from build123d import *

# Parameters (mm, degrees)
BOSS_EXTRU_1_DEPTH      = 5
ESQUISSE12_R            = 3.5
BOSS_EXTRU_2_DEPTH      = 1
ESQUISSE10_RX           = 3.412746185
ESQUISSE10_RY           = 1.923364
ENL_V_MAT_EXTRU_5_DEPTH = 4
ESQUISSE13_R            = 2
ENL_V_MAT_EXTRU_7_DEPTH = 21.846162874
ESQUISSE11_R            = 9.4
ENL_V_MAT_EXTRU_6_DEPTH = 22.060923692


with BuildPart() as part:
    # Esquisse1 → Boss.-Extru.1 (new body)
    with BuildSketch(Plane(origin=(0, 0, 0), x_dir=(1, 0, 0), z_dir=(0, 1, 0))):
        with BuildLine():
            ThreePointArc((-4.625, -8.010734985), (0, -9.25), (4.625, -8.010734985))
            ThreePointArc((4.625, -8.010734985), (9.25, 0), (4.625, 8.010734985))
            ThreePointArc((4.625, 8.010734985), (0, 9.25), (-4.625, 8.010734985))
            ThreePointArc((-4.625, 8.010734985), (-9.25, 0), (-4.625, -8.010734985))
        make_face()
    extrude(amount=BOSS_EXTRU_1_DEPTH)

    # Esquisse8 → Révolution1 (revolve)
    with BuildSketch(Plane.XY, mode=Mode.PRIVATE) as r_volution1_sk:
        Polygon((12.75, 0), (9.25, 0), (9.25, 5), (10.05, 5), align=None)
    revolve(r_volution1_sk.sketch.rotate(Axis((0, 6.978175321, 0), (0, -1, 0)), 90), axis=Axis((0, 6.978175321, 0), (0, -1, 0)))

    # Esquisse12 → Boss.-Extru.2 (add)
    with BuildSketch(Plane.XZ):
        with Locations((0, 12.5)):
            Circle(ESQUISSE12_R)
        with Locations((0, -12.5)):
            Circle(ESQUISSE12_R)
    extrude(amount=-BOSS_EXTRU_2_DEPTH)

    # Esquisse10 → Enlèv. mat.-Extru.5 (cut)
    with BuildSketch(Plane(origin=(0, 5, 0), x_dir=(1, 0, 0), z_dir=(0, 1, 0))):
        with Locations((0, 11.723364)):
            Ellipse(ESQUISSE10_RX, ESQUISSE10_RY)
        with Locations((0, -11.723364)):
            Ellipse(ESQUISSE10_RX, ESQUISSE10_RY)
    extrude(amount=-ENL_V_MAT_EXTRU_5_DEPTH, mode=Mode.SUBTRACT)

    # Esquisse13 → Enlèv. mat.-Extru.7 (cut, through all)
    with BuildSketch(Plane(origin=(0, 1, 0), x_dir=(1, 0, 0), z_dir=(0, 1, 0))):
        with Locations(Location((0, 12.5, 0), (0, 0, 270))):
            Circle(ESQUISSE13_R)
        with Locations(Location((0, -12.5, 0), (0, 0, 270))):
            Circle(ESQUISSE13_R)
    extrude(amount=-ENL_V_MAT_EXTRU_7_DEPTH, mode=Mode.SUBTRACT)

    # Esquisse11 → Enlèv. mat.-Extru.6 (cut, through all)
    with BuildSketch(Plane(origin=(0, 5, 0), x_dir=(1, 0, 0), z_dir=(0, 1, 0))):
        with Locations(Location((0, 0, 0), (0, 0, 270))):
            Circle(ESQUISSE11_R)
    extrude(amount=-ENL_V_MAT_EXTRU_6_DEPTH, mode=Mode.SUBTRACT)


solid = part.part
For this review, take the finished solid that the model builds, in its own axes (mm). A direction names the side the tool comes from. Give positions to 0.01 mm unless a question says otherwise; leave off trailing zeros. One line per question, with ' | ' between items.
1) For faces 3 (the flat face through (2, 1, 14)), 4 (the flat face through (0, 1, -15)), 5 (the cylindrical face through (-1.2, 0.5, -14.1)), list the 3-axis set-ups (+Z, -Z, +X, -X, +Y, -Y) from which the entire face can be reached by the end or side of a thin tool; tool diameter is ignored.
Resolved:
face 3: +Z, +Y | face 4: -Z, +Y | face 5: +Y, -Y
2) Insertion check: pin 1 Ø2 at (x, z) = (6, 11) entering from +Y; pin 2 Ø1.9 at (x, z) = (0, -14) entering from +Y; pin 3 Ø3 at (x, y) = (5.5, 2) entering from +Z; pin 4 Ø6 at (x, z) = (3, -7.5) entering from +Y. Each pin has a flat end and moves straight along its axis. Give the tip position at first contact, or say it passes through.
Resolved:
pin 1: stops at y = 2.26 | pin 2: stops at y = 1 | pin 3: stops at z = 11.43 | pin 4: stops at y = 5
3) To check wall thickness, follow probe 1 along Z at (x, y) = (1, 0.65); probe 2 along X at (y, z) = (0.5, 12.5); probe 3 along X at (y, z) = (1.65, 0). State the ranges of each line that lie inside material, in increasing order.
Resolved:
probe 1: z = -15.85 to -14.23, -10.77 to -9.35, 9.35 to 10.77, 14.23 to 15.85 | probe 2: x = -3.5 to -2, 2 to 3.5 | probe 3: x = -11.86 to -9.4, 9.4 to 11.86
4) The part is to be moulded in two halves that separate along Z. For faces 1 (the flat face through (-8, 0, -6)), 2 (the cylindrical face through (-1.2, 0.5, 10.9)), say which applies: +Z half, -Z half, draft (parallel to the pull), parting line (faces both ways), or undercut.
Resolved:
face 1: draft | face 2: undercut
5) We need section A-A (x = 0). Give the number of separate pieces and of enclosed holes in the cut face, plus the area to 3 significant figures.
Resolved:
separate pieces: 4 | enclosed holes: 0 | area: 8.40 mm2
